Part print with two shaded views. Sizes in mm from the minimum x, y, z corner. A direction names the side the tool comes from. Coordinates: 2 decimals unless noted, no trailing zeros. Loops run counter-clockwise (first coordinate to the right, second up) from the corner with the lowest first, then second, coordinate; pieces in that order, holes last. Notation, with made-up numbers: (-35.5, 51) - (-17.5, 51) arc R8 cw to (-17.5, 57) - close; hole circle Ø10 at (16, 85.5). An arc over 180 degrees is marked (long way). Answer as CSV lines item,"result".
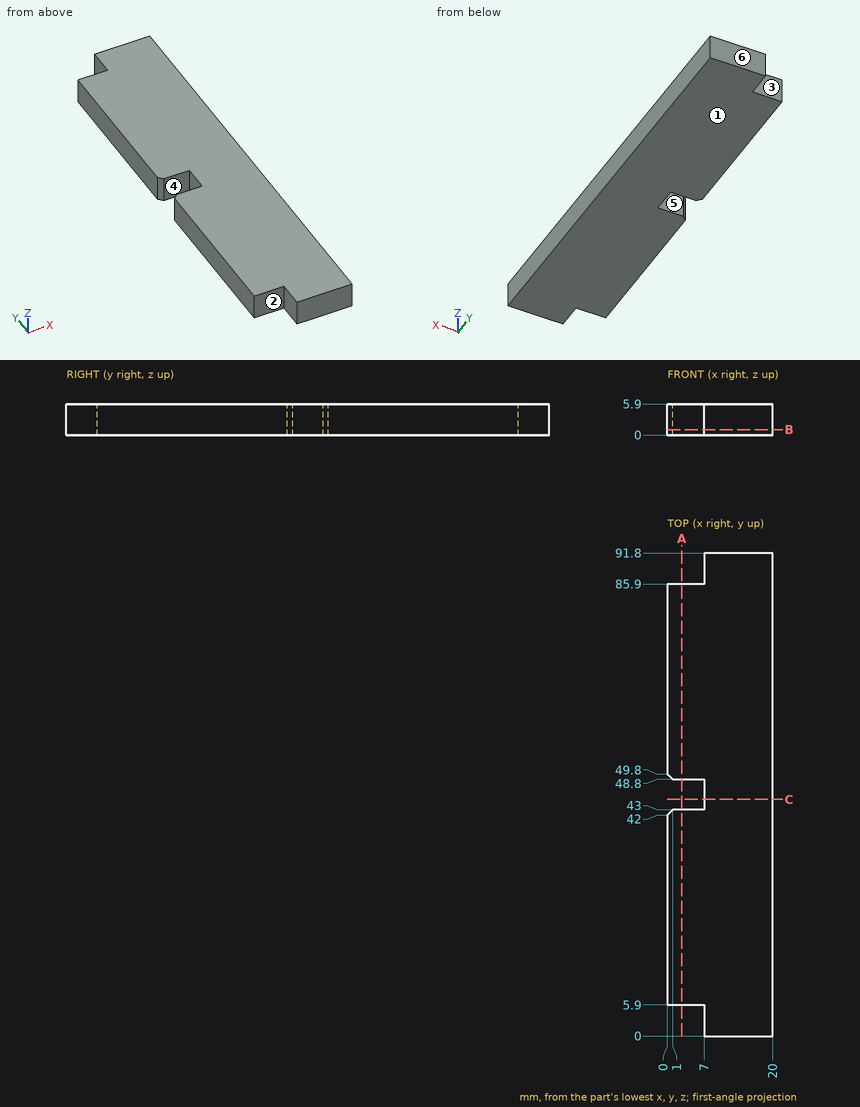
Q1. Which spindle directions (+Z, -Z, +X, -X, +Y, -Y) get a long thin tool onto all of the face, cutting with end or side? Do the marked faces 5 and 6. Say none if no direction does.
Results:
face 5,"+Z, -Z, -X"
face 6,"+Z, -Z, +X, -X, +Y"
Q2. Saw through at C-C (y = 45). Give the cut face in (x, z).
Results:
outline,"(7, 0) - (20, 0) - (20, 5.9) - (7, 5.9) - close"
Q3. Wall check: L1, parallel to Y at x = 5, z = 1.5; L2, parallel to X at y = 45.5, z = 0.6; L3, parallel to X at y = 42.5, z = 5.65. Give the ranges that are in metal, low to high.
Results:
L1,"y = 5.9 to 43, 48.8 to 85.9"
L2,"x = 7 to 20"
L3,"x = 0.5 to 20"
Q4. Flat gauge pins, fed straight in: pin 1 (3 mm diameter, centred on x = 3.5, z = 1.5, fed in from +Y); pin 2 (3 mm diameter, centred on x = 4, z = 3.5, fed in from -Y). Where does each tip first touch, or does it go through?
Results:
pin 1,"stops at y = 85.9"
pin 2,"stops at y = 5.9"
Q5. Saw through at B-B (z = 1.05). Give the cut face in (x, y).
Results:
outline,"(0, 5.9) - (7, 5.9) - (7, 0) - (20, 0) - (20, 91.8) - (7, 91.8) - (7, 85.9) - (0, 85.9) - (0, 49.8) - (1, 48.8) - (7, 48.8) - (7, 43) - (1, 43) - (0, 42) - close"
Q6. Saw through at A-A (x = 2.75). Give the cut face in (y, z), then the cut area to 3 significant figures.
Results:
outline,"(5.9, 0) - (43, 0) - (43, 5.9) - (5.9, 5.9) - close; (48.8, 0) - (85.9, 0) - (85.9, 5.9) - (48.8, 5.9) - close"
area,"438 mm^2"
Q7. Two-plate mould, pull along Y, no slides. Class the marked faces 1, 2, 3 and 4: released by +Y, released by -Y, zero draft, split by the parting line, or undercut.
Results:
face 1,"zero draft"
face 2,"released by -Y"
face 3,"released by +Y"
face 4,"undercut"
